Source: three-view drawing plus pictorial views. Frame: mm from the lowest corner of the part. A direction names the side the tool comes from. Coordinates: 2 decimals unless noted, no trailing zeros. Order: outer loops, then holes, each group sorted by start corner. A loop starts at its lowest first (then second) coordinate and runs counter-clockwise, first axis right, second up. Notation, with made-up numbers: (-5, 23) -> (3, 23) arc R21 ccw to (3, 38) -> close; hole circle Ø3 at (47.25, -26). An arc over 180 degrees is marked (long way). Use one line per item in the form item = value. Start each with the question number.
1) Ray query, line 1 along X through (y, z) = (10, 45); line 2 along X through (y, z) = (5.5, 18) (1 decimal); line 3 along Z through (x, y) = (49.5, 15). Return the intervals inside material, ascending.
2) Pin query (flat end, axial travel): pin 1 (10 mm diameter, centred on y = 26, z = 6.5, fed in from -X); pin 2 (8 mm diameter, centred on x = 15.5, z = 11.5, fed in from +Y); pin 3 (12.5 mm diameter, centred on y = 10.5, z = 29.5, fed in from +X); pin 4 (3 mm diameter, centred on x = 52.5, y = 19.5, fed in from +Z). Return the tip coordinate at first contact, or that it passes through.
3) Access query for the marked faces 1, 2 and 3. Directions: +Z, -Z, +X, -X, +Y, -Y. A direction counts if a zero-diameter tool reaches every point of the face in a straight line with its end or side. Return the directions, or none.
4) Section query D-D on y = 39.5. Output: boundary loops of the cut face in (x, z).
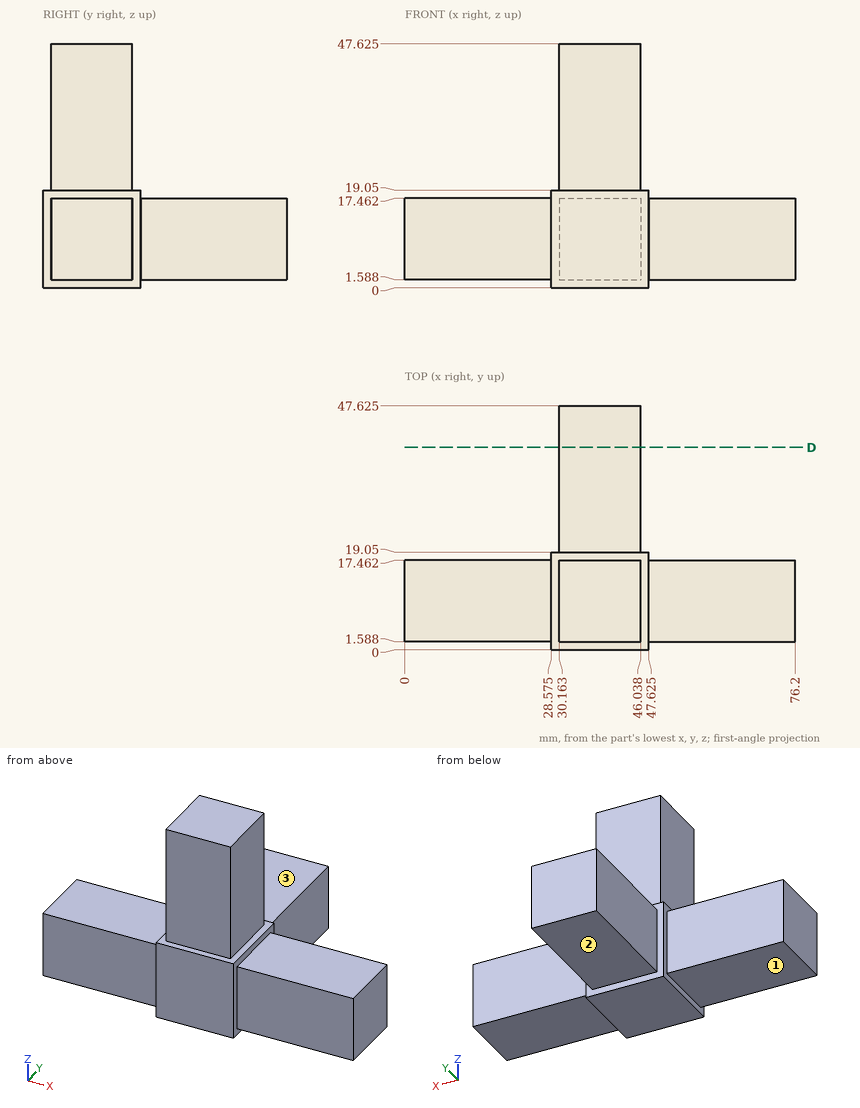
Answers below:
q1.line_1 = 30.16 to 46.04
q1.line_2 = 28.6 to 47.6
q1.line_3 = 1.59 to 17.46
q2.pin_1 = 30.16
q2.pin_2 = 17.46
q2.pin_3 = 46.04
q2.pin_4 = through
q3.face_1 = -Z, -X, +Y, -Y
q3.face_2 = -Z, +X, -X, +Y
q3.face_3 = +Z, +X, -X, +Y
q4.outline = (30.16, 1.59) -> (46.04, 1.59) -> (46.04, 17.46) -> (30.16, 17.46) -> close
